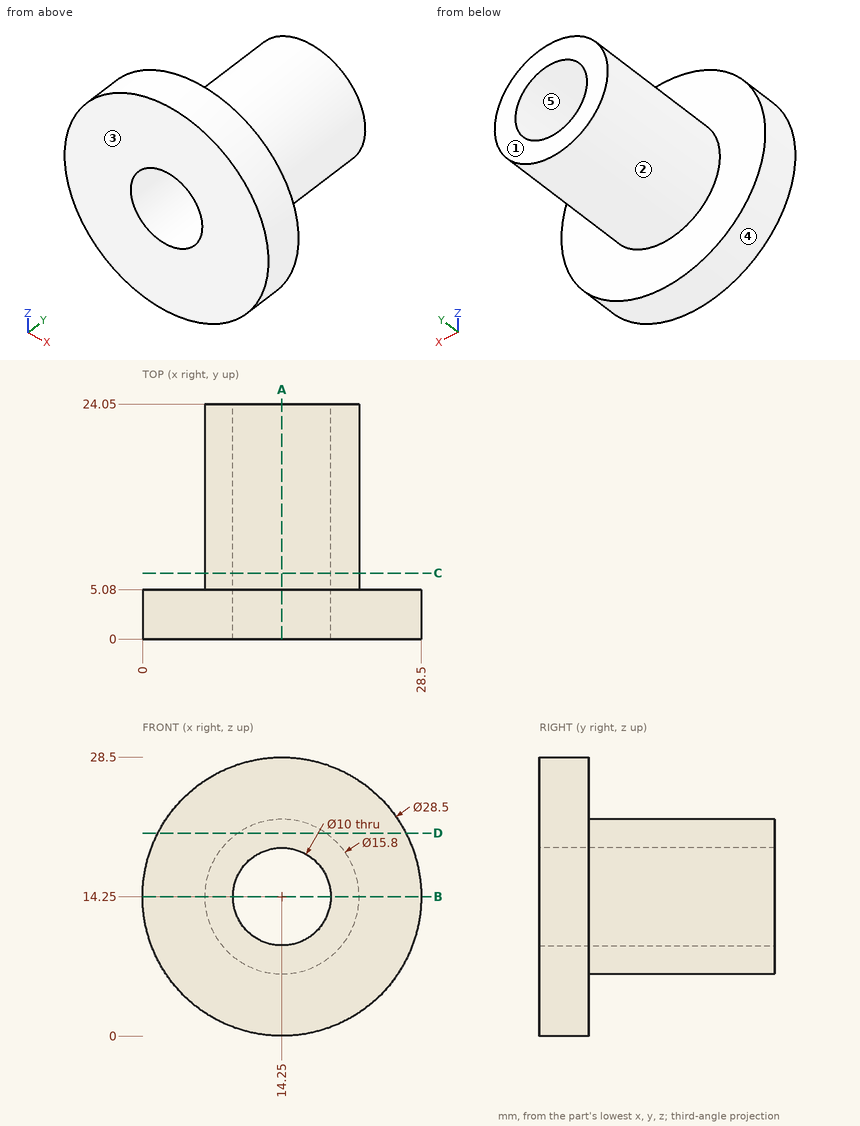
Job drawing, mm, ordinate dimensions from the low corner. One solid piece. A direction names the side the tool comes from. Coordinates: 2 decimals unless noted, no trailing zeros. Write each loop counter-clockwise with the first axis right and the second up, starting at its lowest first coordinate (ties: lowest second). Pieces come first, ordered by that corner, then holes. Notation, with made-up numbers: M -18.75,24.25 L -9.75,24.25 A21 ccw -9.75,60.25 Z; hole C 4.25,20 d6. An arc over 180 degrees is marked long. Answer as a JSON object with one key per item and string values. Group by question number.
1) Tool access for the marked faces 1 and 2: list every direction of +Z, -Z, +X, -X, +Y, -Y with a clear straight run to the whole face (end or side of a thin tool).
2) Mould opens along Z. For the marked faces 3, 4 and 5 say: +Z half, -Z half, draft (parallel to the pull), parting line (faces both ways), or undercut.
3) Saw through at A-A (x = 14.25). Write the cut outline in (y, z), plus the area to 3 significant figures.
4) Pin check, flat tips, straight feed: pin 1 Ø1.5 at (y, z) = (16, 20.5) entering from +X; pin 2 Ø4 at (y, z) = (9, 20) entering from +X; pin 3 Ø2 at (y, z) = (5, 20) entering from +X (3 decimals). Stop position of each tip, or through.
5) Saw through at B-B (z = 14.25). Write the cut outline in (x, y), plus the area to 3 significant figures.
6) Saw through at D-D (z = 20.75). Write the cut outline in (x, y).
7) Saw through at C-C (y = 6.75). Write the cut outline in (x, z).
8) Wall check: line 1 (X direction, y = 12.5, z = 14.25); line 2 (Y direction, x = 5.5, z = 7.5); line 3 (X direction, y = 16, z = 18.5). Give the ranges that are in metal, low to high. Write a range as from..to.
Values follow:
{
 "1": {"face 1": "+Z, -Z, +X, -X, +Y", "face 2": "+Y"},
 "2": {"face 3": "draft", "face 4": "parting line", "face 5": "undercut"},
 "3": {"outline": "M 0,0 L 5.08,0 L 5.08,6.35 L 24.05,6.35 L 24.05,9.25 L 0,9.25 Z; M 0,19.25 L 24.05,19.25 L 24.05,22.15 L 5.08,22.15 L 5.08,28.5 L 0,28.5 Z", "area": "204 mm2"},
 "4": {"pin 1": "stops at x = 19.92", "pin 2": "stops at x = 21.2", "pin 3": "stops at x = 27.685"},
 "5": {"outline": "M 0,0 L 9.25,0 L 9.25,24.05 L 6.35,24.05 L 6.35,5.08 L 0,5.08 Z; M 19.25,0 L 28.5,0 L 28.5,5.08 L 22.15,5.08 L 22.15,24.05 L 19.25,24.05 Z", "area": "204 mm2"},
 "6": {"outline": "M 1.57,0 L 26.93,0 L 26.93,5.08 L 18.74,5.08 L 18.74,24.05 L 9.76,24.05 L 9.76,5.08 L 1.57,5.08 Z"},
 "7": {"outline": "C 14.25,14.25 d15.8; hole C 14.25,14.25 d10"},
 "8": {"line 1": "x = 6.35..9.25, 19.25..22.15", "line 2": "y = 0..5.08", "line 3": "x = 7.59..11.62, 16.88..20.91"}
}
